Geometry check sheet. Reference: the model listing, model coordinates, mm. A direction names the side the tool comes from. Round coordinates to 2 decimals unless told otherwise and drop trailing zeros. Write each loop counter-clockwise with the first axis right and the second up, starting at its lowest first coordinate (ties: lowest second). Pieces come first, ordered by that corner, then holes. Notation, with made-up numbers: M 73,-27 L 96,-27 A14 ccw 96,-22 Z; hole C 89,70 d8. An arc over 180 degrees is marked long. One line per item, written item: value. Start each with the question number.
1. Scan lines: probe 1 along X at (y, z) = (-36.5, 228.5); probe 2 along Z at (x, y) = (364.5, -21.5); probe 3 along X at (y, z) = (-52, 193.5). Record each from-to range of solid material in increasing order. Write a range as [from, to].
2. Access from +Z, -Z, +X, -X, +Y, -Y to the whole of each face (thin tool, end or side, straight path). Record for faces 4 (the flat face through (356.6, 0, 590.3)), 5 (the flat face through (10, -34, 291)), 6 (the flat face through (717, -37, 600)), 7 (the flat face through (1777.121, -34.017, 299.394)), 8 (the flat face through (1668.355, -36.975, 209.517)).
3. Section check A-A (y = -30.5). Record the boundary of the cut face in (x, z).
4. Section check B-B (z = 282.5). Record the boundary of the cut face in (x, y).
5. Depth check by flat-ended pin: P1, Ø22.5, axis at x = 534.5, y = -49, coming from the -Z side; P2, Ø3, axis at x = 1419.5, y = -49.5, coming from the +Z side; P3, Ø6, axis at y = -57.5, z = 69, coming from the +X side. Enter the tip coordinate at first touch or a pass-through.
6. Release check for a two-part mould opening along X. For faces 1 (the flat face through (715, -34, 460)), 2 (the flat face through (75, -71, 0)), 3 (the flat face through (1797.785, -36.975, 295.8)) record: pulls with the +X half, pulls with the -X half, needs draft (parallel to the pull), parting line crosses it, or undercut.
7. Section check D-D (z = 370). Record the boundary of the cut face in (x, y).
8. Section check C-C (x = 1300.5). Record the boundary of the cut face in (y, z), and give its area (3 significant figures).
from build123d import *

# Parameters (mm, degrees)
F1_DEPTH = 75
F3_DEPTH = 69


with BuildPart() as f1:
    # F0 (on Front) → F1 (new body)
    with BuildSketch(Plane.XZ):
        Polygon((0, 600), (0, 0), (150, 0), (150, 450), (1265, 450), (1265, 0), (1415, 0), (1415, 413.248549), (1928.905491, 0), (2170, 0), (1415, 600), align=None)
    extrude(amount=F1_DEPTH)

    # F2 (on face) → F3 (cut)
    with BuildSketch(Plane(origin=(0, 0, 0), x_dir=(-1, 0, 0), z_dir=(0, 1, 0))):
        Polygon((-1405, 0), (-1275, 0), (-1275, 460), (-140, 460), (-140, 0), (-10, 0), (-10, 590), (-1410.821319, 590.520203), (-2153.822899, 0), (-1938.905491, 0), (-1405, 429.331216), align=None)
    extrude(amount=-F3_DEPTH, mode=Mode.SUBTRACT)


solid = f1.part
Result sheet:
1. probe 1: x = [0, 10], [140, 150], [1265, 1275], [1405, 1415], [1644.75, 1654.75], [1866.32, 1882.47]
1. probe 2: z = [450, 460], [590.13, 600]
1. probe 3: x = [0, 10], [140, 150], [1265, 1275], [1405, 1415], [1688.27, 1698.27], [1910.36, 1926.51]
2. face 4: +Z, -Z, +X, -X, +Y
2. face 5: -Z, +Y
2. face 6: +Z, +X, -X, +Y, -Y
2. face 7: +Y
2. face 8: -Z, +Y, -Y
3. outline: M 0,0 L 10,0 L 10,590 L 1410.82,590.52 L 2153.82,0 L 2170,0 L 1415,600 L 0,600 Z; M 140,0 L 150,0 L 150,450 L 1265,450 L 1265,0 L 1275,0 L 1275,460 L 140,460 Z; M 1405,0 L 1415,0 L 1415,413.25 L 1928.91,0 L 1938.91,0 L 1405,429.33 Z
4. outline: M 0,-75 L 150,-75 L 150,0 L 140,0 L 140,-69 L 10,-69 L 10,0 L 0,0 Z; M 1265,-75 L 1415,-75 L 1415,0 L 1405,0 L 1405,-69 L 1275,-69 L 1275,0 L 1265,0 Z; M 1577.6,-75 L 1814.52,-75 L 1814.52,0 L 1798.38,0 L 1798.38,-69 L 1587.6,-69 L 1587.6,0 L 1577.6,0 Z
5. P1: stops at z = 450
5. P2: stops at z = 597.62
5. P3: stops at x = 2086.95
6. face 1: undercut
6. face 2: needs draft
6. face 3: pulls with the +X half
7. outline: M 0,-75 L 150,-75 L 150,0 L 140,0 L 140,-69 L 10,-69 L 10,0 L 0,0 Z; M 1265,-75 L 1415,-75 L 1415,0 L 1405,0 L 1405,-69 L 1275,-69 L 1275,0 L 1265,0 Z; M 1468.78,-75 L 1704.42,-75 L 1704.42,0 L 1688.28,0 L 1688.28,-69 L 1478.78,-69 L 1478.78,0 L 1468.78,0 Z
8. outline: M -75,0 L -69,0 L -69,590.48 L 0,590.48 L 0,600 L -75,600 Z
8. area: 4,260 mm2
